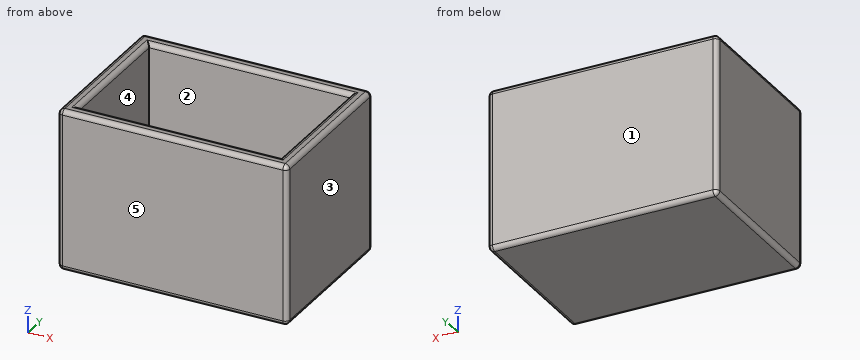
```python
from build123d import *

# Parameters (mm, degrees)
F0_W     = 12.7
F0_H     = 8.89
F1_DEPTH = 8.89
F2_T     = -0.762
F3_R     = 0.254
F4_R     = 0.254


with BuildPart() as f1:
    # F0 (on Top) → F1 (new body)
    with BuildSketch(Plane.XY):
        with Locations((-41.3615499459, 30.1495660652)):
            Rectangle(F0_W, F0_H)
    extrude(amount=F1_DEPTH)

    # F2
    f2_openings = [f1.faces().sort_by_distance(p)[0] for p in [
        (-41.36155, 30.149566, 8.89),
    ]]
    offset(amount=F2_T, openings=f2_openings)

    # F3
    f3_edges = [f1.edges().sort_by_distance(p)[0] for p in [
        (-41.36155, 33.832566, 8.89),
        (-41.36155, 25.704566, 8.89),
        (-41.36155, 26.466566, 8.89),
        (-41.36155, 34.594566, 8.89),
        (-46.94955, 30.149566, 8.89),
        (-47.71155, 30.149566, 8.89),
        (-35.77355, 30.149566, 8.89),
        (-35.01155, 30.149566, 8.89),
        (-35.01155, 25.704566, 4.445),
        (-47.71155, 25.704566, 4.445),
        (-47.71155, 34.594566, 4.445),
        (-35.01155, 34.594566, 4.445),
        (-35.01155, 30.149566, 0),
        (-41.36155, 25.704566, 0),
        (-47.71155, 30.149566, 0),
        (-41.36155, 34.594566, 0),
    ]]
    fillet(f3_edges, radius=F3_R)

    # F4
    f4_edges = [f1.edges().sort_by_distance(p)[0] for p in [
        (-41.36155, 33.832566, 0.762),
        (-35.77355, 30.149566, 0.762),
        (-41.36155, 26.466566, 0.762),
        (-46.94955, 30.149566, 0.762),
    ]]
    fillet(f4_edges, radius=F4_R)


solid = f1.part
```
Model file for the job. Use its own axes, mm. Face numbers are marked on the shaded views. A direction names the side the tool comes from. Coordinates: 2 decimals unless noted, no trailing zeros. Loops run counter-clockwise (first coordinate to the right, second up) from the corner with the lowest first, then second, coordinate; pieces in that order, holes last. Notation, with made-up numbers: M 14.25,20.5 L 69.25,20.5 A27 cw 69.25,49.5 Z; hole C 9.25,0.5 d8. An arc over 180 degrees is marked long. Use CSV: the item, a comma, the result in double quotes. Start each with the question number.
1. Probe probe 1 along X at (y, z) = (33.5, 2); probe 2 along Y at (x, z) = (-38.5, 5.75); probe 3 along Z at (x, y) = (-38.5, 33.5). List the from-to ranges inside material, lowest first. Write a range as [from, to].
2. Two-plate mould, pull along X, no slides. Class the marked faces 1, 2 and 3: pulls with the +X half, pulls with the -X half, needs draft (parallel to the pull), parting line crosses it, or undercut.
3. Tool access for the marked faces 4 and 5: list every direction of +Z, -Z, +X, -X, +Y, -Y with a clear straight run to the whole face (end or side of a thin tool).
4. Band-saw the part on B-B, the plane x = -42.25. List the corners of the cut face in (y, z).
5. Band-saw the part on A-A, the plane z = 6.5. List the corners of the cut face in (x, y).
6. Flat gauge pin, fed straight in: pin 1 (1 mm diameter, centred on x = -46, y = 32.5, fed in from +Z). Where does the tip first touch, or does it go through?
7. Band-saw the part on C-C, the plane y = 30. List the corners of the cut face in (x, z).
Entries:
1,probe 1,"x = [-47.71, -46.95], [-35.77, -35.01]"
1,probe 2,"y = [25.7, 26.47], [33.83, 34.59]"
1,probe 3,"z = [0, 0.76]"
2,face 1,"needs draft"
2,face 2,"undercut"
2,face 3,"pulls with the +X half"
3,face 4,"+Z"
3,face 5,"+Z, -Z, +X, -X, -Y"
4,outline,"M 25.7,0.25 A0.25 ccw 25.96,0 L 34.34,0 A0.25 ccw 34.59,0.25 L 34.59,8.64 A0.25 ccw 34.34,8.89 L 34.09,8.89 A0.25 ccw 33.83,8.64 L 33.83,1.02 A0.25 cw 33.58,0.76 L 26.72,0.76 A0.25 cw 26.47,1.02 L 26.47,8.64 A0.25 ccw 26.21,8.89 L 25.96,8.89 A0.25 ccw 25.7,8.64 Z"
5,outline,"M -47.71,25.96 A0.25 ccw -47.46,25.7 L -35.27,25.7 A0.25 ccw -35.01,25.96 L -35.01,34.34 A0.25 ccw -35.27,34.59 L -47.46,34.59 A0.25 ccw -47.71,34.34 Z; hole M -46.95,26.47 L -35.77,26.47 L -35.77,33.83 L -46.95,33.83 Z"
6,pin 1,"stops at z = 0.76"
7,outline,"M -47.71,0.25 A0.25 ccw -47.46,0 L -35.27,0 A0.25 ccw -35.01,0.25 L -35.01,8.64 A0.25 ccw -35.27,8.89 L -35.52,8.89 A0.25 ccw -35.77,8.64 L -35.77,1.02 A0.25 cw -36.03,0.76 L -46.7,0.76 A0.25 cw -46.95,1.02 L -46.95,8.64 A0.25 ccw -47.2,8.89 L -47.46,8.89 A0.25 ccw -47.71,8.64 Z"
